Source: three-view drawing plus pictorial views. Frame: mm from the lowest corner of the part. Round coordinates to 2 decimals unless told otherwise and drop trailing zeros. Loops run counter-clockwise (first coordinate to the right, second up) from the corner with the lowest first, then second, coordinate; pieces in that order, holes last. Notation, with made-up numbers: M 47,75.5 L 91,75.5 A32 ccw 91,108.5 Z; hole C 21,80 d8. An arc over 180 degrees is marked long. Return JSON: item names as keys, results as strings. Group by question number.
1) Section D-D (y = 35). Output: boundary loops of the cut face in (x, z).
2) Material intervals for line 1 (Y direction, x = 12.5, z = 67.5); line 2 (X direction, y = 265, z = 28); line 3 (Y direction, x = 10.25, z = 15.5), sorted ascending. Write a range as from..to.
3) Contact query for flat-ended pins moving along their axis: P1, Ø10, axis at x = 22, z = 62, coming from the -Y side; P2, Ø5, axis at x = 12.5, y = 150, coming from the +Z side. Output: stop coordinate, or through.
4) Section C-C (x = 12.5). Output: boundary loops of the cut face in (y, z), plus the area to 4 significant figures.
5) Section B-B (z = 84). Output: boundary loops of the cut face in (x, y), plus the area to 3 significant figures.
6) Section A-A (y = 150). Output: boundary loops of the cut face in (x, z), plus the area to 3 significant figures.
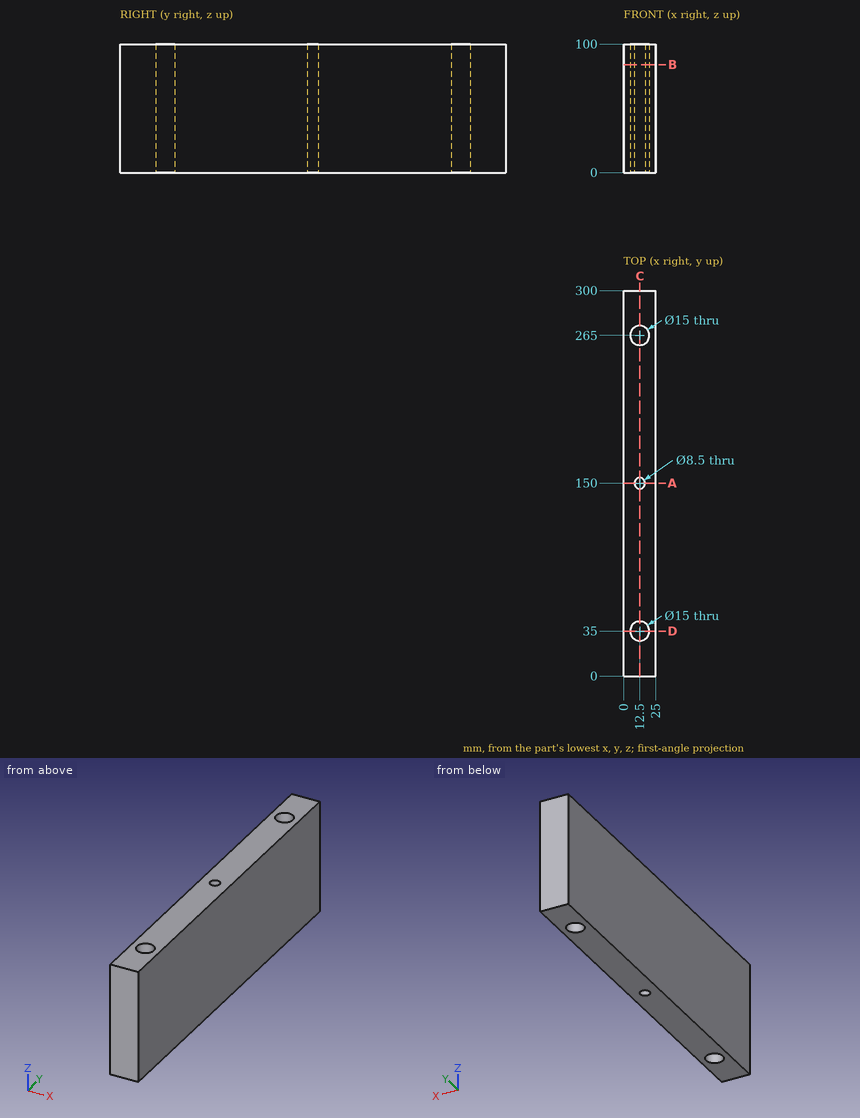
Returned:
{
 "1": {"outline": "M 0,0 L 5,0 L 5,100 L 0,100 Z; M 20,0 L 25,0 L 25,100 L 20,100 Z"},
 "2": {"line 1": "y = 0..27.5, 42.5..145.75, 154.25..257.5, 272.5..300", "line 2": "x = 0..5, 20..25", "line 3": "y = 0..27.85, 42.15..146.39, 153.61..257.85, 272.15..300"},
 "3": {"P1": "stops at y = 0", "P2": "passes through"},
 "4": {"outline": "M 0,0 L 27.5,0 L 27.5,100 L 0,100 Z; M 42.5,0 L 145.75,0 L 145.75,100 L 42.5,100 Z; M 154.25,0 L 257.5,0 L 257.5,100 L 154.25,100 Z; M 272.5,0 L 300,0 L 300,100 L 272.5,100 Z", "area": "26,150 mm^2"},
 "5": {"outline": "M 0,0 L 25,0 L 25,300 L 0,300 Z; hole C 12.5,35 d15; hole C 12.5,265 d15; hole C 12.5,150 d8.5", "area": "7,090 mm^2"},
 "6": {"outline": "M 0,0 L 8.25,0 L 8.25,100 L 0,100 Z; M 16.75,0 L 25,0 L 25,100 L 16.75,100 Z", "area": "1,650 mm^2"}
}
